from build123d import *

# Parameters (mm, degrees)
SKETCH028_R           = 2
PAD011_DEPTH          = 1.05
POCKET023_DEPTH       = 71.792855
POLARPATTERN_COUNT    = 4
POCKET024_DEPTH       = 71.792855
POLARPATTERN001_COUNT = 4
PAD012_DEPTH          = 0.75


with BuildPart() as part:
    # Sketch028 → Pad011 (new body)
    with BuildSketch(Plane.YZ):
        with BuildLine():
            Line((-12.5, 9.5), (-12.5, -9.5))
            ThreePointArc((-12.5, -9.5), (-11.62132, -11.62132), (-9.5, -12.5))
            Line((-9.5, -12.5), (9.5, -12.5))
            ThreePointArc((9.5, -12.5), (11.62132, -11.62132), (12.5, -9.5))
            Line((12.5, -9.5), (12.5, 9.5))
            ThreePointArc((12.5, 9.5), (11.62132, 11.62132), (9.5, 12.5))
            Line((9.5, 12.5), (-9.5, 12.5))
            ThreePointArc((-9.5, 12.5), (-11.62132, 11.62132), (-12.5, 9.5))
        make_face()
        Circle(SKETCH028_R, mode=Mode.SUBTRACT)
    extrude(amount=PAD011_DEPTH)

    # Sketch029 (on Face11 of Pad011) → Pocket023 (cut, through all)
    with BuildSketch(Plane.YZ.offset(1.05)):
        with BuildLine():
            ThreePointArc((1.362563, 3.760774), (0, 4), (-1.362563, 3.760774))
            ThreePointArc((-2.214165, 6.111258), (-2.963606, 4.510215), (-1.362563, 3.760774))
            ThreePointArc((2.214165, 6.111258), (0, 6.5), (-2.214165, 6.111258))
            ThreePointArc((1.362563, 3.760774), (2.963606, 4.510215), (2.214165, 6.111258))
        make_face()
    pocket023 = extrude(amount=-POCKET023_DEPTH, mode=Mode.SUBTRACT)

    # PolarPattern: Pocket023 ×4 about axis
    polarpattern_axis = Axis((1.05, 0, 0), (1, 0, 0))
    for i in range(1, POLARPATTERN_COUNT):
        add(pocket023.rotate(polarpattern_axis, i * 360 / POLARPATTERN_COUNT), mode=Mode.SUBTRACT)

    # Sketch030 (on Face5 of PolarPattern) → Pocket024 (cut, through all)
    with BuildSketch(Plane.YZ.offset(1.05)):
        with BuildLine():
            ThreePointArc((-1.955695, 8.271956), (-6.010408, 6.010408), (-8.271956, 1.955695))
            ThreePointArc((-10.704884, 2.5309), (-9.776022, 1.026833), (-8.271956, 1.955695))
            ThreePointArc((-2.5309, 10.704884), (-7.778175, 7.778175), (-10.704884, 2.5309))
            ThreePointArc((-1.955695, 8.271956), (-1.026833, 9.776022), (-2.5309, 10.704884))
        make_face()
    pocket024 = extrude(amount=-POCKET024_DEPTH, mode=Mode.SUBTRACT)

    # PolarPattern001: Pocket024 ×4 about axis
    polarpattern001_axis = Axis((1.05, 0, 0), (1, 0, 0))
    for i in range(1, POLARPATTERN001_COUNT):
        add(pocket024.rotate(polarpattern001_axis, i * 360 / POLARPATTERN001_COUNT), mode=Mode.SUBTRACT)

    # Sketch031 (on Face5 of PolarPattern001) → Pad012 (join)
    with BuildSketch(Plane.YZ.offset(1.05)):
        with BuildLine():
            Line((-12.5, 9.5), (-12.5, -9.5))
            ThreePointArc((-12.5, -9.5), (-11.62132, -11.62132), (-9.5, -12.5))
            Line((-9.5, -12.5), (9.5, -12.5))
            ThreePointArc((9.5, -12.5), (11.62132, -11.62132), (12.5, -9.5))
            Line((12.5, -9.5), (12.5, 9.5))
            ThreePointArc((12.5, 9.5), (11.62132, 11.62132), (9.5, 12.5))
            Line((9.5, 12.5), (-9.5, 12.5))
            ThreePointArc((-9.5, 12.5), (-11.62132, 11.62132), (-12.5, 9.5))
        make_face()
        with BuildLine():
            Line((-11.7, 9.5), (-11.7, -9.5))
            ThreePointArc((-11.7, -9.5), (-11.055635, -11.055635), (-9.5, -11.7))
            Line((-9.5, -11.7), (9.5, -11.7))
            ThreePointArc((9.5, -11.7), (11.055635, -11.055635), (11.7, -9.5))
            Line((11.7, -9.5), (11.7, 9.5))
            ThreePointArc((11.7, 9.5), (11.055635, 11.055635), (9.5, 11.7))
            Line((9.5, 11.7), (-9.5, 11.7))
            ThreePointArc((-9.5, 11.7), (-11.055635, 11.055635), (-11.7, 9.5))
        make_face(mode=Mode.SUBTRACT)
    extrude(amount=PAD012_DEPTH)


with BuildPart() as part_1:
    # Body009 placement: moved
    add(part.part.moved(Location((4.85, 35.05, 22.7))))


solid = part_1.part
Verification items for the finished model (mm, model axes). A direction names the side the tool comes from. Round coordinates to 2 decimals unless told otherwise and drop trailing zeros. Loops run counter-clockwise (first coordinate to the right, second up) from the corner with the lowest first, then second, coordinate; pieces in that order, holes last. Notation, with made-up numbers: (84.25, -13) - (136.25, -13) arc R28 cw to (136.25, 16) - close; hole circle Ø5 at (62.5, -17). An arc over 180 degrees is marked (long way). Use one line per item in the form item = value.
1. Scan lines: probe 1 along Z at (x, y) = (5.65, 35.05); probe 2 along Z at (x, y) = (6.05, 29.5); probe 3 along Z at (x, y) = (5.2, 25.25). Record each from-to range of solid material in increasing order.
A:
probe_1 = 10.2 to 16.2, 18.7 to 20.7, 24.7 to 26.7, 29.2 to 35.2
probe_2 = 10.2 to 11, 34.4 to 35.2
probe_3 = 10.22 to 17.7, 21.67 to 23.73, 27.7 to 35.18
2. Draft check along Y on faces 4 (the cylindrical face through (5.382, 32.096, 18.216)), 5 (the flat face through (6, 22.55, 23)), 6 (the flat face through (4.85, 35, 26)). Enter one of: pulls with the +Y half, pulls with the -Y half, needs draft (parallel to the pull), parting line crosses it, or undercut.
A:
face_4 = undercut
face_5 = pulls with the -Y half
face_6 = needs draft
3. Section check A-A on z = 22.7. Record the cut outline in (x, y), and give its area (3 significant figures).
A:
outline = (4.85, 22.55) - (6.65, 22.55) - (6.65, 23.35) - (5.9, 23.35) - (5.9, 28.55) - (4.85, 28.55) - close; (4.85, 31.05) - (5.9, 31.05) - (5.9, 33.05) - (4.85, 33.05) - close; (4.85, 37.05) - (5.9, 37.05) - (5.9, 39.05) - (4.85, 39.05) - close; (4.85, 41.55) - (5.9, 41.55) - (5.9, 46.75) - (6.65, 46.75) - (6.65, 47.55) - (4.85, 47.55) - close
area = 18.0 mm²
4. Section check D-D on z = 30. Record the cut outline in (x, y).
A:
outline = (4.85, 22.55) - (6.65, 22.55) - (6.65, 23.35) - (5.9, 23.35) - (5.9, 26.82) - (4.85, 26.82) - close; (4.85, 30.7) - (5.9, 30.7) - (5.9, 39.4) - (4.85, 39.4) - close; (4.85, 43.28) - (5.9, 43.28) - (5.9, 46.75) - (6.65, 46.75) - (6.65, 47.55) - (4.85, 47.55) - close
5. Section check B-B on y = 35.05. Record the cut outline in (x, z), and give its area (3 significant figures).
A:
outline = (4.85, 10.2) - (6.65, 10.2) - (6.65, 11) - (5.9, 11) - (5.9, 16.2) - (4.85, 16.2) - close; (4.85, 18.7) - (5.9, 18.7) - (5.9, 20.7) - (4.85, 20.7) - close; (4.85, 24.7) - (5.9, 24.7) - (5.9, 26.7) - (4.85, 26.7) - close; (4.85, 29.2) - (5.9, 29.2) - (5.9, 34.4) - (6.65, 34.4) - (6.65, 35.2) - (4.85, 35.2) - close
area = 18.0 mm²
6. Access from +Z, -Z, +X, -X, +Y, -Y to the whole of each face (thin tool, end or side, straight path). Record for faces 1 (the cylindrical face through (5.382, 42.888, 30.418)), 2 (the flat face through (5.9, 35, 25)), 3 (the flat face through (6.65, 35, 10.7)).
A:
face_1 = +X, -X
face_2 = +X
face_3 = +Z, -Z, +X, +Y, -Y
7. Section check C-C on y = 44.25. Record the cut outline in (x, z), and give its area (3 significant figures).
A:
outline = (4.85, 10.2) - (6.65, 10.2) - (6.65, 11) - (5.9, 11) - (5.9, 16.67) - (4.85, 16.67) - close; (4.85, 21.67) - (5.9, 21.67) - (5.9, 23.73) - (4.85, 23.73) - close; (4.85, 28.73) - (5.9, 28.73) - (5.9, 34.4) - (6.65, 34.4) - (6.65, 35.2) - (4.85, 35.2) - close
area = 16.9 mm²
8. Gauge pin test, flat end, axial feed: pin 1 Ø1.5 at (y, z) = (34.5, 26) entering from +X. Record the tip position at first contact, or that the pin passes through.
A:
pin_1 = 5.9
